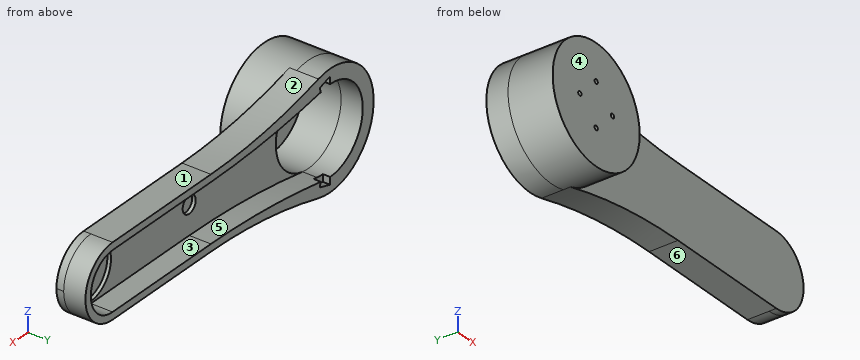
```python
from build123d import *

# Parameters (mm, degrees)
BOSS_EXTRUDE1_DEPTH     = 15
SKETCH2_R               = 40
SKETCH2_R_2             = 30
BOSS_EXTRUDE2_DEPTH     = 25.8
SKETCH3_R               = 40
BOSS_EXTRUDE3_DEPTH     = 5
SKETCH4_R               = 6
SKETCH4_R_2             = 18.5
BOSS_EXTRUDE4_DEPTH     = 5
SKETCH6_R               = 6
SKETCH6_R_2             = 18.5
BOSS_EXTRUDE5_DEPTH     = 2.5
CUT_EXTRUDE1_DEPTH      = 5
SKETCH8_R               = 1.5
CUT_EXTRUDE2_DEPTH      = 1
CUT_EXTRUDE2_DEPTH_BACK = 46.8


with BuildPart() as part:
    # Sketch1 → Boss-Extrude1 (new body)
    with BuildSketch(Plane(origin=(0, 0, 0), x_dir=(1, 0, 0), z_dir=(0, 1, 0))):
        with BuildLine():
            ThreePointArc((200, -25), (225, 0), (200, 25))
            Line((200, 25), (109.6, 25))
            ThreePointArc((109.6, 25), (59.713041879, 28.397959328), (10.747591761, 38.529070471))
            ThreePointArc((10.747591761, 38.529070471), (-40, 0), (10.747591761, -38.529070471))
            ThreePointArc((10.747591761, -38.529070471), (59.713041879, -28.397959328), (109.6, -25))
            Line((109.6, -25), (200, -25))
        make_face()
        with BuildLine():
            Line((109.6, 20), (200, 20))
            ThreePointArc((200, 20), (220, 0), (200, -20))
            Line((200, -20), (109.6, -20))
            ThreePointArc((109.6, -20), (57.298273937, -22.381082353), (5.429254567, -29.504630058))
            ThreePointArc((5.429254567, -29.504630058), (-30, 0), (5.429254567, 29.504630058))
            ThreePointArc((5.429254567, 29.504630058), (57.298273937, 22.381082353), (109.6, 20))
        make_face(mode=Mode.SUBTRACT)
    extrude(amount=BOSS_EXTRUDE1_DEPTH)

    # Sketch2 → Boss-Extrude2 (add)
    with BuildSketch(Plane.XZ):
        Circle(SKETCH2_R)
        Circle(SKETCH2_R_2, mode=Mode.SUBTRACT)
    extrude(amount=BOSS_EXTRUDE2_DEPTH)

    # Sketch3 → Boss-Extrude3 (add)
    with BuildSketch(Plane.XZ.offset(25.8)):
        Circle(SKETCH3_R)
    extrude(amount=BOSS_EXTRUDE3_DEPTH)

    # Sketch4 → Boss-Extrude4 (add)
    with BuildSketch(Plane.XZ):
        with BuildLine():
            ThreePointArc((185, -20), (175, 0), (185, 20))
            Line((185, 20), (109.6, 20))
            ThreePointArc((109.6, 20), (70.154992453, 21.353125364), (30.895437645, 25.406139666))
            ThreePointArc((30.895437645, 25.406139666), (37.655129171, 13.494118982), (40, 0))
            ThreePointArc((40, 0), (37.655129171, -13.494118982), (30.895437645, -25.406139666))
            ThreePointArc((30.895437645, -25.406139666), (70.154992453, -21.353125364), (109.6, -20))
            Line((109.6, -20), (185, -20))
        make_face()
        with Locations((109.6, 0)):
            Circle(SKETCH4_R, mode=Mode.SUBTRACT)
        with BuildLine():
            Line((200, 20), (185, 20))
            ThreePointArc((185, 20), (175, 0), (185, -20))
            Line((185, -20), (200, -20))
            ThreePointArc((200, -20), (220, 0), (200, 20))
        make_face()
        with Locations((200, 0)):
            Circle(SKETCH4_R_2, mode=Mode.SUBTRACT)
        with BuildLine():
            ThreePointArc((225, 0), (217.67766953, 17.67766953), (200, 25))
            ThreePointArc((200, 25), (192.09430585, 23.717082451), (185, 20))
            Line((185, 20), (200, 20))
            ThreePointArc((200, 20), (220, 0), (200, -20))
            Line((200, -20), (185, -20))
            ThreePointArc((185, -20), (192.09430585, -23.717082451), (200, -25))
            ThreePointArc((200, -25), (217.67766953, -17.67766953), (225, 0))
        make_face()
        with BuildLine():
            ThreePointArc((185, 20), (192.09430585, 23.717082451), (200, 25))
            Line((200, 25), (109.6, 25))
            ThreePointArc((109.6, 25), (59.713041879, 28.397959328), (10.747591761, 38.529070471))
            ThreePointArc((10.747591761, 38.529070471), (21.830902473, 33.51733428), (30.895437645, 25.406139666))
            ThreePointArc((30.895437645, 25.406139666), (70.154992453, 21.353125364), (109.6, 20))
            Line((109.6, 20), (185, 20))
        make_face()
        with BuildLine():
            Line((109.6, -25), (200, -25))
            ThreePointArc((200, -25), (192.09430585, -23.717082451), (185, -20))
            Line((185, -20), (109.6, -20))
            ThreePointArc((109.6, -20), (70.154992453, -21.353125364), (30.895437645, -25.406139666))
            ThreePointArc((30.895437645, -25.406139666), (21.830902473, -33.51733428), (10.747591761, -38.529070471))
            ThreePointArc((10.747591761, -38.529070471), (59.713041879, -28.397959328), (109.6, -25))
        make_face()
    extrude(amount=BOSS_EXTRUDE4_DEPTH)

    # Sketch6 → Boss-Extrude5 (add)
    with BuildSketch(Plane.XZ.offset(5)):
        with Locations((109.6, 0)):
            Circle(SKETCH6_R)
        with Locations((200, 0)):
            Circle(SKETCH6_R_2)
    extrude(amount=-BOSS_EXTRUDE5_DEPTH)

    # Sketch7 → Cut-Extrude1 (cut)
    with BuildSketch(Plane(origin=(0, 15, 0), x_dir=(1, 0, 0), z_dir=(0, 1, 0))):
        with BuildLine():
            ThreePointArc((5.429254567, -29.504630058), (2.725903361, -29.875900838), (0, -30))
            Line((0, -30), (0, -35))
            Line((0, -35), (9.583148475, -32.142857143))
            Line((9.583148475, -32.142857143), (8.624081591, -28.926049021))
            ThreePointArc((8.624081591, -28.926049021), (7.026260133, -29.213086928), (5.429254567, -29.504630058))
        make_face()
        with BuildLine():
            Line((0, 35), (0, 30))
            ThreePointArc((0, 30), (2.725903361, 29.875900838), (5.429254567, 29.504630058))
            ThreePointArc((5.429254567, 29.504630058), (7.026260133, 29.213086928), (8.624081591, 28.926049021))
            Line((8.624081591, 28.926049021), (9.583148475, 32.142857143))
            Line((9.583148475, 32.142857143), (0, 35))
        make_face()
    extrude(amount=-CUT_EXTRUDE1_DEPTH, mode=Mode.SUBTRACT)

    # Sketch8 → Cut-Extrude2 (cut, two sides)
    with BuildSketch(Plane.XZ.offset(30.8)) as cut_extrude2_sk:
        with Locations((0, 15)):
            Circle(SKETCH8_R)
        with Locations((15, 0)):
            Circle(SKETCH8_R)
        with Locations((0, -15)):
            Circle(SKETCH8_R)
        with Locations((-15, 0)):
            Circle(SKETCH8_R)
    extrude(amount=CUT_EXTRUDE2_DEPTH, mode=Mode.SUBTRACT)
    extrude(cut_extrude2_sk.sketch, amount=-CUT_EXTRUDE2_DEPTH_BACK, mode=Mode.SUBTRACT)


solid = part.part
```
The listing builds one solid part. Answer for the finished solid, in the listing's coordinates (mm). Face numbers are marked on the shaded views. A direction names the side the tool comes from. Give positions to 0.01 mm unless a question says otherwise; leave off trailing zeros. Write each loop counter-clockwise with the first axis right and the second up, starting at its lowest first coordinate (ties: lowest second). Pieces come first, ordered by that corner, then holes. Notation, with made-up numbers: M -15.5,70 L -6.5,70 A35 cw -6.5,109 Z; hole C -29.5,34 d2. An arc over 180 degrees is marked long. Write each question's results on one line, items separated by ' | '.
Q1. Section D-D, the plane y = -18.5 is taken. Write down the section's boundary in (x, z).
Output values:
outline: C 0,0 d80; hole C 0,0 d60
Q2. Section C-C, the plane x = 47 is taken. Write down the section's boundary in (y, z), then the cut area to 3 significant figures.
Output values:
outline: M -5,-30.36 L 15,-30.36 L 15,-23.41 L 0,-23.41 L 0,23.41 L 15,23.41 L 15,30.36 L -5,30.36 Z | area: 512 mm2
Q3. A tool of negligible diameter and unlimited length cuts with its end or side. For the marked faces 4, 5 and 6, from which of +Z, -Z, +X, -X, +Y, -Y can it reach the whole face along a straight path? Write none if from no direction.
Output values:
face 4: +Z, -Z, +X, -X, -Y | face 5: +Y | face 6: -Z, +X, +Y, -Y
Q4. Flat-ended cylindrical pins translate along their axes: P1, Ø2, axis at x = 18, z = -9.5, coming from the +Y side; P2, Ø5, axis at y = 5, z = -14.5, coming from the +X side; P3, Ø2, axis at y = -20.5, z = -14, coming from the -X side. Find the tip coordinate at first contact, or state that the pin passes through.
Output values:
P1: y = -25.8 | P2: x = 221.93 | P3: x = -37.83
Q5. Consider L1, parallel to Z at x = 0, y = -26.9; L2, parallel to Z at x = 109.6, y = -1.1; L3, parallel to Z at x = 200, y = -1. Determine where each line is inside the solid, lowest interval first. Write a range as from..to.
Output values:
L1: -40..-16.5, -13.5..13.5, 16.5..40 | L2: -25..-6, 6..25 | L3: -25..-18.5, 18.5..25
Q6. For a pull along X with two mould halves and no side action, classify the marked faces 1, 2 and 3 as released by +X, released by -X, zero draft, split by the parting line, or undercut.
Output values:
face 1: zero draft | face 2: released by +X | face 3: undercut
Q7. Section A-A, the plane y = 6 is taken. Write down the section's boundary in (x, z).
Output values:
outline: M 10.75,-38.53 A367.91 cw 109.6,-25 L 200,-25 A25 ccw 200,25 L 109.6,25 A367.91 cw 10.75,38.53 A40 ccw long Z; hole M 5.43,-29.5 A575.61 cw 109.6,-20 L 200,-20 A20 ccw 200,20 L 109.6,20 A575.61 cw 5.43,29.5 A30 ccw long Z
Q8. Section B-B, the plane x = 173.5 is taken. Write down the section's boundary in (y, z).
Output values:
outline: M -5,-25 L 15,-25 L 15,-20 L 0,-20 L 0,20 L 15,20 L 15,25 L -5,25 Z
